from build123d import *

# Parameters (mm, degrees)
BOSS_EXTRUDE1_DEPTH     = 10
BOSS_EXTRUDE2_START     = 1
SKETCH3_R               = 3
BOSS_EXTRUDE2_DEPTH     = 1
CUT_EXTRUDE1_DEPTH      = 59
CUT_EXTRUDE1_DEPTH_BACK = 104


with BuildPart() as part:
    # Sketch2 → Boss-Extrude1 (new body)
    with BuildSketch(Plane(origin=(0, 0, 0), x_dir=(1, 0, 0), z_dir=(0, 1, 0))):
        with BuildLine():
            ThreePointArc((54.859329632, -46.484559643), (50.497240278, 6.301499085), (-2.28881845, 1.939409731))
            ThreePointArc((-2.28881845, 1.939409731), (-1.939409731, -2.28881845), (2.28881845, -1.939409731))
            ThreePointArc((2.28881845, -1.939409731), (46.618420816, 1.723862186), (50.281692732, -42.605740181))
            ThreePointArc((50.281692732, -42.605740181), (50.631101451, -46.833968361), (54.859329632, -46.484559643))
        make_face()
    extrude(amount=BOSS_EXTRUDE1_DEPTH)

    # Sketch3 → Boss-Extrude2 (add)
    with BuildSketch(Plane.XZ.offset(BOSS_EXTRUDE2_START)):
        with Locations(Location((0, 0, 0), (0, 0, 270))):
            Circle(SKETCH3_R)
    extrude(amount=-BOSS_EXTRUDE2_DEPTH)

    # Sketch4 → Cut-Extrude1 (cut, two sides: drawn at the far end of the back side and taken through both)
    with BuildSketch(Plane.XZ.offset(-CUT_EXTRUDE1_DEPTH_BACK)):
        with BuildLine():
            Line((54.859329632, 46.484559643), (50.281692732, 42.605740181))
            ThreePointArc((50.281692732, 42.605740181), (49.580702363, 44.792219186), (50.631101451, 46.833968361))
            ThreePointArc((50.631101451, 46.833968361), (52.817580456, 47.534958731), (54.859329632, 46.484559643))
        make_face()
    extrude(amount=CUT_EXTRUDE1_DEPTH + CUT_EXTRUDE1_DEPTH_BACK, mode=Mode.SUBTRACT)


solid = part.part
The listing builds one solid part. Answer for the finished solid, in the listing's coordinates (mm). Give positions to 0.01 mm unless a question says otherwise; leave off trailing zeros. Loops run counter-clockwise (first coordinate to the right, second up) from the corner with the lowest first, then second, coordinate; pieces in that order, holes last. Notation, with made-up numbers: (-22, -39.75) - (33, -39.75) arc R25 cw to (33, -27.75) - close; hole circle Ø9 at (45.5, 12.25). An arc over 180 degrees is marked (long way). Use one line per item in the form item = value.
1. Section A-A on x = 0 is taken. Give the vertices of the cut face in (y, z), then the cut area to 3 significant figures.
Calculated:
outline = (-1, -3) - (0, -3) - (0, -4.41) - (10, -4.41) - (10, 3) - (-1, 3) - close
area = 80.1 mm^2
2. The mould has two halves that part along Z. Classify faces 1 (the face through (51.12, 4.93, -5.76)), 2 (the face through (48, 0, -3)), 3 (the face through (46.086, 4.93, -2.165)): pulls with the +Z half, pulls with the -Z half, needs draft (parallel to the pull), parting line crosses it, or undercut.
Calculated:
face_1 = parting line crosses it
face_2 = needs draft
face_3 = undercut
3. Section C-C on y = 1 is taken. Give the vertices of the cut face in (x, z).
Calculated:
outline = (-2.29, -1.94) arc R37.45 ccw to (54.86, 46.48) - (50.28, 42.61) arc R31.45 cw to (2.29, 1.94) arc R3 ccw to start
4. Section D-D on z = 40.5 is taken. Give the vertices of the cut face in (x, y), then the cut area to 3 significant figures.
Calculated:
outline = (51.92, 0) - (59, 0) - (59, 10) - (51.92, 10) - close
area = 70.9 mm^2
5. Section B-B on z = 0 is taken. Give the vertices of the cut face in (x, y).
Calculated:
outline = (-3, -1) - (3, -1) - (3, 0) - (4.08, 0) - (4.08, 10) - (-3, 10) - close; (48.49, 0) - (56.4, 0) - (56.4, 10) - (48.49, 10) - close
6. Find the intervals of material crossed by line 1 along Y through (x, z) = (51, -5); line 2 along X through (y, z) = (4, 2); line 3 along Z through (x, y) = (3, 9.75), in increasing order. Write a range as [from, to].
Calculated:
line_1 = [0, 10]
line_2 = [-2.24, 2.24], [50.33, 57.78]
line_3 = [-7.06, 1.13]
7. Given pin 1 Ø3 at (y, z) = (4, 38) entering from +X; pin 2 Ø4 at (y, z) = (1, 14.5) entering from +X; pin 3 Ø1 at (x, y) = (46.5, 4.5) entering from -Z, each flat-ended and moving along its own axis, determine where each tip first touches the part or whether it passes through.
Calculated:
pin_1 = 60.93
pin_2 = 63.29
pin_3 = -9.57
